from build123d import *

# Parameters (mm, degrees)
F0_R     = 1.5
F0_R_2   = 14.5
F1_DEPTH = 4
F2_R     = 12
F0_R_3   = 12.4
F3_DEPTH = 6
F4_DEPTH = 16


with BuildPart() as f1:
    # F0 (on Top) → F1 (new body)
    with BuildSketch(Plane.XY):
        with BuildLine():
            Line((-50, 40.1261364576), (-50, -40.1261364576))
            ThreePointArc((-50, -40.1261364576), (-48.5323223277, -39.658202653), (-47, -39.5))
            Line((-47, -39.5), (-47, 39.5))
            ThreePointArc((-47, 39.5), (-48.5323223277, 39.658202653), (-50, 40.1261364576))
        make_face()
        with BuildLine():
            Line((-50, -50), (-40.1261364576, -50))
            ThreePointArc((-40.1261364576, -50), (-39.658202653, -48.5323223277), (-39.5, -47))
            Line((-39.5, -47), (-47, -47))
            Line((-47, -47), (-47, -39.5))
            ThreePointArc((-47, -39.5), (-48.5323223277, -39.658202653), (-50, -40.1261364576))
            Line((-50, -40.1261364576), (-50, -50))
        make_face()
        with BuildLine():
            Line((-47, -47), (-39.5, -47))
            ThreePointArc((-39.5, -47), (-41.6966991411, -41.6966991411), (-47, -39.5))
            Line((-47, -39.5), (-47, -47))
        make_face()
        with Locations((-44, -44)):
            Circle(F0_R, mode=Mode.SUBTRACT)
        with BuildLine():
            Line((-40.1261364576, -50), (40.1261364576, -50))
            ThreePointArc((40.1261364576, -50), (39.658202653, -48.5323223277), (39.5, -47))
            Line((39.5, -47), (-39.5, -47))
            ThreePointArc((-39.5, -47), (-39.658202653, -48.5323223277), (-40.1261364576, -50))
        make_face()
        with BuildLine():
            Line((40.1261364576, -50), (50, -50))
            Line((50, -50), (50, -40.1261364576))
            ThreePointArc((50, -40.1261364576), (48.5323223277, -39.658202653), (47, -39.5))
            Line((47, -39.5), (47, -47))
            Line((47, -47), (39.5, -47))
            ThreePointArc((39.5, -47), (39.658202653, -48.5323223277), (40.1261364576, -50))
        make_face()
        with BuildLine():
            ThreePointArc((47, -39.5), (41.6966991411, -41.6966991411), (39.5, -47))
            Line((39.5, -47), (47, -47))
            Line((47, -47), (47, -39.5))
        make_face()
        with Locations((44, -44)):
            Circle(F0_R, mode=Mode.SUBTRACT)
        with BuildLine():
            ThreePointArc((47, -39.5), (48.5323223277, -39.658202653), (50, -40.1261364576))
            Line((50, -40.1261364576), (50, 40.1261364576))
            ThreePointArc((50, 40.1261364576), (48.5323223277, 39.658202653), (47, 39.5))
            Line((47, 39.5), (47, -39.5))
        make_face()
        with BuildLine():
            ThreePointArc((47, 39.5), (48.5323223277, 39.658202653), (50, 40.1261364576))
            Line((50, 40.1261364576), (50, 50))
            Line((50, 50), (40.1261364576, 50))
            ThreePointArc((40.1261364576, 50), (39.658202653, 48.5323223277), (39.5, 47))
            Line((39.5, 47), (47, 47))
            Line((47, 47), (47, 39.5))
        make_face()
        with BuildLine():
            ThreePointArc((39.5, 47), (41.6966991411, 41.6966991411), (47, 39.5))
            Line((47, 39.5), (47, 47))
            Line((47, 47), (39.5, 47))
        make_face()
        with Locations((44, 44)):
            Circle(F0_R, mode=Mode.SUBTRACT)
        with BuildLine():
            ThreePointArc((39.5, 47), (39.658202653, 48.5323223277), (40.1261364576, 50))
            Line((40.1261364576, 50), (-40.1261364576, 50))
            ThreePointArc((-40.1261364576, 50), (-39.658202653, 48.5323223277), (-39.5, 47))
            Line((-39.5, 47), (39.5, 47))
        make_face()
        with BuildLine():
            Line((-50, 50), (-50, 40.1261364576))
            ThreePointArc((-50, 40.1261364576), (-48.5323223277, 39.658202653), (-47, 39.5))
            Line((-47, 39.5), (-47, 47))
            Line((-47, 47), (-39.5, 47))
            ThreePointArc((-39.5, 47), (-39.658202653, 48.5323223277), (-40.1261364576, 50))
            Line((-40.1261364576, 50), (-50, 50))
        make_face()
        with BuildLine():
            Line((-47, 47), (-47, 39.5))
            ThreePointArc((-47, 39.5), (-41.6966991411, 41.6966991411), (-39.5, 47))
            Line((-39.5, 47), (-47, 47))
        make_face()
        with Locations((-44, 44)):
            Circle(F0_R, mode=Mode.SUBTRACT)
        with BuildLine():
            Line((-39.5, -47), (39.5, -47))
            ThreePointArc((39.5, -47), (41.6966991411, -41.6966991411), (47, -39.5))
            Line((47, -39.5), (47, 39.5))
            ThreePointArc((47, 39.5), (41.6966991411, 41.6966991411), (39.5, 47))
            Line((39.5, 47), (-39.5, 47))
            ThreePointArc((-39.5, 47), (-41.6966991411, 41.6966991411), (-47, 39.5))
            Line((-47, 39.5), (-47, -39.5))
            ThreePointArc((-47, -39.5), (-41.6966991411, -41.6966991411), (-39.5, -47))
        make_face()
        Circle(F0_R_2, mode=Mode.SUBTRACT)
    extrude(amount=F1_DEPTH)

    # F2
    f2_edges = [f1.edges().sort_by_distance(p)[0] for p in [
        (-50, 50, 2),
        (50, 50, 2),
        (50, -50, 2),
        (-50, -50, 2),
    ]]
    fillet(f2_edges, radius=F2_R)

    # F0 (on Top) → F3 (join)
    with BuildSketch(Plane.XY):
        Circle(F0_R_2)
        Circle(F0_R_3, mode=Mode.SUBTRACT)
    extrude(amount=F3_DEPTH)

    # F0 (on Top) → F4 (join)
    with BuildSketch(Plane.XY):
        Circle(F0_R_3)
    extrude(amount=F4_DEPTH)


solid = f1.part
Here's how the part is built. I have some questions about the finished solid (model axes, mm). A direction names the side the tool comes from. Round coordinates to 2 decimals unless told otherwise and drop trailing zeros. Write each loop counter-clockwise with the first axis right and the second up, starting at its lowest first coordinate (ties: lowest second). Pieces come first, ordered by that corner, then holes.
1. I need wall thicknesses on L1, parallel to Y at x = 44, z = 2.85; L2, parallel to Z at x = -8.5, y = -31; L3, parallel to Y at x = 7, z = 10.25. Which ranges of each line are inside material? Lowest first, please.
2. Will these pins go through, and if not, where does the flat tip stop? pin 1 Ø5 at (x, y) = (-44, -44) entering from +Z; pin 2 Ø1.8 at (x, y) = (44, -44) entering from +Z; pin 3 Ø2 at (x, z) = (-9, 6) entering from -Y.
3. For faces 4 (the flat face through (11, 7, 6)), 5 (the cylindrical face through (42.8, 43.1, 2)), which set-ups out of +Z, -Z, +X, -X, +Y, -Y let a thin tool reach every point of the face, with its end or its side?
4. Suppose I cut it at B-B (x = -44). List the corners of the cut face in (y, z) for me, and give its area (3 significant figures).
5. Suppose I cut it at C-C (y = 0). List the corners of the cut face in (x, z) for me, and give its area (3 significant figures).
6. If we mould it in two halves opening along Y, with no side actions, what happens to faces 1 (the flat face through (50, -1, 2)), 2 (the cylindrical face through (46.39, -46.58, 2.03)), 3 (the cylindrical face through (42.8, -44.9, 2))? For each: released by +Y, released by -Y, zero draft, split by the parting line, or undercut.
7. Suppose I cut it at A-A (z = 2.75). List the corners of the cut face in (x, y) for me, and give its area (3 significant figures).
Answer sheet:
1. L1: y = -48.39 to -45.5, -42.5 to 42.5, 45.5 to 48.39
1. L2: z = 0 to 4
1. L3: y = -10.24 to 10.24
2. pin 1: stops at z = 4
2. pin 2: passes through
2. pin 3: stops at y = -12.09
3. face 4: +Z
3. face 5: +Z, -Z
4. outline: (-48.39, 0) - (-45.5, 0) - (-45.5, 4) - (-48.39, 4) - close; (-42.5, 0) - (42.5, 0) - (42.5, 4) - (-42.5, 4) - close; (45.5, 0) - (48.39, 0) - (48.39, 4) - (45.5, 4) - close
4. area: 363 mm2
5. outline: (-50, 0) - (50, 0) - (50, 4) - (14.5, 4) - (14.5, 6) - (12.4, 6) - (12.4, 16) - (-12.4, 16) - (-12.4, 6) - (-14.5, 6) - (-14.5, 4) - (-50, 4) - close
5. area: 706 mm2
6. face 1: zero draft
6. face 2: released by -Y
6. face 3: undercut
7. outline: (-50, -38) arc R12 ccw to (-38, -50) - (38, -50) arc R12 ccw to (50, -38) - (50, 38) arc R12 ccw to (38, 50) - (-38, 50) arc R12 ccw to (-50, 38) - close; hole circle Ø3 at (-44, -44); hole circle Ø3 at (-44, 44); hole circle Ø3 at (44, -44); hole circle Ø3 at (44, 44)
7. area: 9,850 mm2
